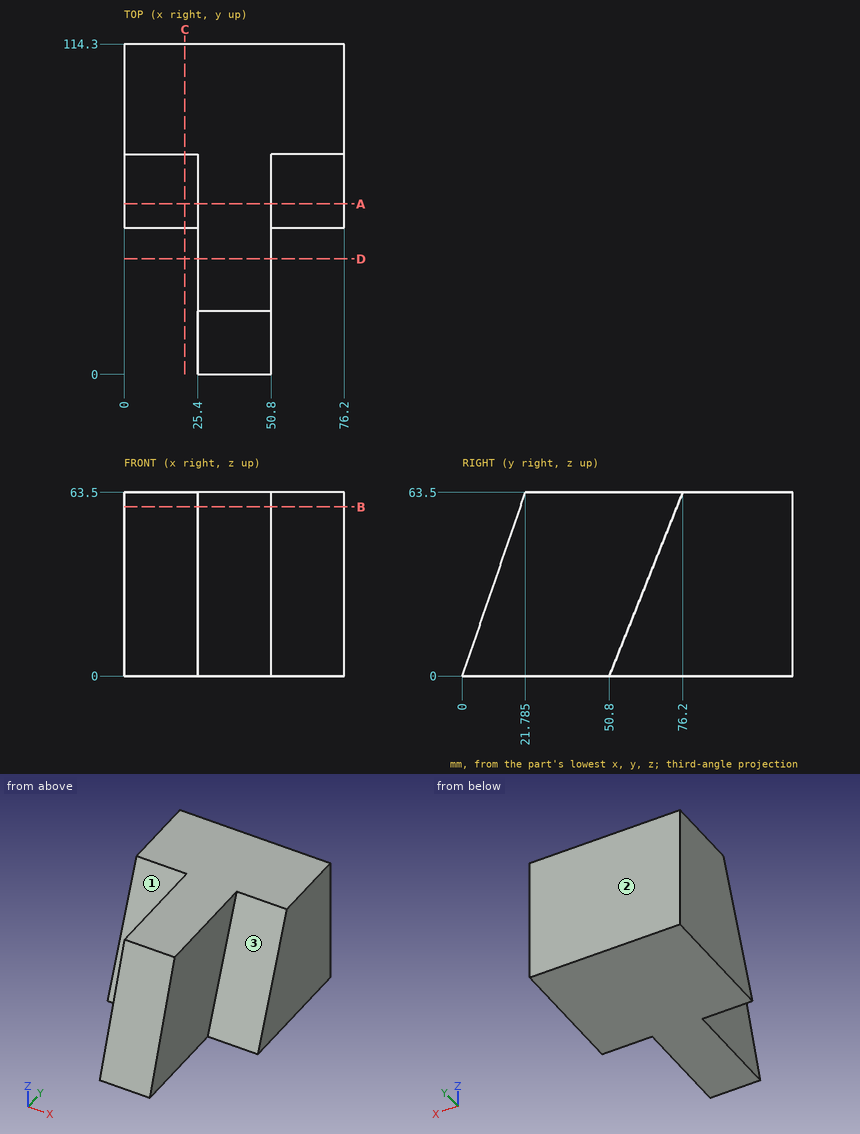
Source: three-view drawing plus pictorial views. Frame: mm from the lowest corner of the part. A direction names the side the tool comes from. Round coordinates to 2 decimals unless told otherwise and drop trailing zeros. Write each loop counter-clockwise with the first axis right and the second up, starting at its lowest first coordinate (ties: lowest second). Pieces come first, ordered by that corner, then holes. Notation, with made-up numbers: (89, 41.25) -> (124, 41.25) arc R31 cw to (124, 69.25) -> close; hole circle Ø5 at (26.5, -24). An arc over 180 degrees is marked (long way). Return JSON: item names as keys, results as strings.
Q1. Section D-D on y = 40. Return the cut outline in (x, z).
From the geometry:
{"outline": "(25.4, 0) -> (50.8, 0) -> (50.8, 63.5) -> (25.4, 63.5) -> close"}
Q2. Section C-C on x = 21. Return the cut outline in (y, z).
From the geometry:
{"outline": "(50.8, 0) -> (114.3, 0) -> (114.3, 63.5) -> (76.2, 63.5) -> close"}
Q3. Section B-B on z = 58.5. Return the cut outline in (x, y).
From the geometry:
{"outline": "(0, 74.2) -> (25.4, 74.2) -> (25.4, 20.07) -> (50.8, 20.07) -> (50.8, 74.2) -> (76.2, 74.2) -> (76.2, 114.3) -> (0, 114.3) -> close"}
Q4. Set-up query: the marked faces 1, 2 and 3. Return all of +Z, -Z, +X, -X, +Y, -Y with unobstructed straight access to the full face (end or side cutting, diameter ignored); none if empty.
From the geometry:
{"face 1": "+Z, -X, -Y", "face 2": "+Z, -Z, +X, -X, +Y", "face 3": "+Z, +X, -Y"}
Q5. Section A-A on y = 59. Return the cut outline in (x, z), and give its area (3 significant figures).
From the geometry:
{"outline": "(0, 0) -> (76.2, 0) -> (76.2, 20.5) -> (50.8, 20.5) -> (50.8, 63.5) -> (25.4, 63.5) -> (25.4, 20.5) -> (0, 20.5) -> close", "area": "2,650 mm2"}
Q6. Ray query, line 1 (X direction, y = 43, z = 21); line 2 (Y direction, x = 55, z = 14); line 3 (Y direction, x = 15.5, z = 24.5). Return the intervals inside material, ascending.
From the geometry:
{"line 1": "25.4 to 50.8", "line 2": "56.4 to 114.3", "line 3": "60.6 to 114.3"}
Q7. First-contact query: pin 1 Ø1 at (y, z) = (15, 17) entering from +X; pin 2 Ø6 at (y, z) = (51.5, 34.5) entering from -X. Flat tips, straight axial feed; report the tip coordinate or a pass-through.
From the geometry:
{"pin 1": "x = 50.8", "pin 2": "x = 25.4"}
